Source: CAD feature listing. Evaluate the final solid. Frame: model axes, mm. Give positions to 0.01 mm unless a question says otherwise; leave off trailing zeros. Order: outer loops, then holes, each group sorted by start corner. A loop starts at its lowest first (then second) coordinate and runs counter-clockwise, first axis right, second up.
from build123d import *

# Parameters (mm, degrees)
ESQUISSE1_R                  = 4.1
ESQUISSE1_R_2                = 2.1
BOSS_EXTRU_1_DEPTH           = 6
ESQUISSE2_R                  = 17.5
BOSS_EXTRU_3_DEPTH           = 10
CONG_5_R                     = 0.5
R_P_TITION_CIRCULAIRE2_COUNT = 5
CONG_6_R                     = 0.5
ENL_V_MAT_EXTRU_1_DEPTH      = 1


with BuildPart() as part:
    # Esquisse1 → Boss.-Extru.1 (new body)
    with BuildSketch(Plane.XY):
        Circle(ESQUISSE1_R)
        Circle(ESQUISSE1_R_2, mode=Mode.SUBTRACT)
    extrude(amount=BOSS_EXTRU_1_DEPTH)

    # Esquisse2 → Boss.-Extru.3 (add)
    with BuildSketch(Plane.XY.offset(6)):
        Circle(ESQUISSE2_R)
        with BuildLine():
            Line((2, 3.579106034), (2, 15.370426149))
            ThreePointArc((2, 15.370426149), (0, -15.5), (-2, 15.370426149))
            Line((-2, 15.370426149), (-2, 3.579106034))
            ThreePointArc((-2, 3.579106034), (0, -4.1), (2, 3.579106034))
        make_face(mode=Mode.SUBTRACT)
        with BuildLine():
            Line((-0.5, 4.06939799), (-0.5, 15.491933385))
            ThreePointArc((-0.5, 15.491933385), (0, 15.5), (0.5, 15.491933385))
            Line((0.5, 15.491933385), (0.5, 4.06939799))
            ThreePointArc((0.5, 4.06939799), (0, 4.1), (-0.5, 4.06939799))
        make_face(mode=Mode.SUBTRACT)
    boss_extru_3 = extrude(amount=BOSS_EXTRU_3_DEPTH)

    # Congé5
    # the kernel refuses this fillet: 0.5 mm, written as the material it adds along each edge
    with BuildSketch(Plane(origin=(2, 3.579106034, 6), x_dir=(0.856640365534706, -0.5159140278540265, 0), z_dir=(0, 0, 1))) as cong_5_piece_1:
        with BuildLine():
            CenterArc((0.282708153, 0.499735946), CONG_5_R, 211.058569469, 57.079265472)
            Line((-0.14561203, 0.241778932), (0, 0))
            ThreePointArc((0, 0), (0.133230279, 0.002165243), (0.266460558, 0))
        make_face()
    extrude(amount=10)
    with BuildSketch(Plane(origin=(2, 15.370426149, 6), x_dir=(0, -1, 0), z_dir=(0, 0, 1))) as cong_5_piece_2:
        with BuildLine():
            CenterArc((0.580226691, 0.5), CONG_5_R, 170.405931773, 99.594068227)
            ThreePointArc((0.087220043, 0.583333333), (0.040835089, 0.292081575), (0, 0))
            Line((0, 0), (0.580226691, 0))
        make_face()
    extrude(amount=10)
    with BuildSketch(Plane(origin=(-2, 15.370426149, 6), x_dir=(0, -1, 0), z_dir=(0, 0, 1))) as cong_5_piece_3:
        with BuildLine():
            CenterArc((0.580226691, -0.5), CONG_5_R, 90, 99.594068227)
            ThreePointArc((0.087220043, -0.583333333), (0.040835089, -0.292081575), (0, 0))
            Line((0, 0), (0.580226691, 0))
        make_face()
    extrude(amount=10)
    with BuildSketch(Plane(origin=(-2, 3.579106034, 6), x_dir=(-0.8566403655347238, -0.515914027853997, 0), z_dir=(0, 0, 1))) as cong_5_piece_4:
        with BuildLine():
            CenterArc((0.282708153, -0.499735946), CONG_5_R, 91.862165059, 57.079265472)
            Line((-0.14561203, -0.241778932), (0, 0))
            ThreePointArc((0, 0), (0.133230279, -0.002165243), (0.266460558, 0))
        make_face()
    extrude(amount=10)

    # Répétition circulaire2: Boss.-Extru.3 ×5 about axis
    r_p_tition_circulaire2_axis = Axis((0, 0, 0), (0, 0, 1))
    for i in range(1, R_P_TITION_CIRCULAIRE2_COUNT):
        add(boss_extru_3.rotate(r_p_tition_circulaire2_axis, i * 360 / R_P_TITION_CIRCULAIRE2_COUNT))

    # Congé6
    # the kernel refuses this fillet: 0.5 mm, written as the material it adds along each edge
    with BuildSketch(Plane(origin=(-14.000109958, 6.651835923, 6), x_dir=(0.95105651629517, -0.3090169943748974, 0), z_dir=(0, 0, 1)), Plane(origin=(-10.652543801, -11.259365461, 6), x_dir=(0.5877852522924284, 0.8090169943749799, 0), z_dir=(0, 0, 1)), Plane(origin=(7.416475823, -13.61050647, 6), x_dir=(-0.5877852522925181, 0.8090169943749146, 0), z_dir=(0, 0, 1)), Plane(origin=(15.236177936, 2.847609858, 6), x_dir=(-0.9510565162951373, -0.30901699437499736, 0), z_dir=(0, 0, 1))) as cong_6_piece_1:
        with BuildLine():
            CenterArc((0.580226691, 0.5), CONG_6_R, 170.405931773, 99.594068227)
            ThreePointArc((0.087220043, 0.583333333), (0.040835089, 0.292081575), (0, 0))
            Line((0, 0), (0.580226691, 0))
        make_face()
    extrude(amount=10)
    with BuildSketch(Plane(origin=(-4.021966105, -0.796108444, 6), x_dir=(-0.9510565162951476, 0.30901699437496566, 0), z_dir=(0, 0, 1)), Plane(origin=(-0.485711754, -4.07112811, 6), x_dir=(-0.587785252292492, -0.8090169943749336, 0), z_dir=(0, 0, 1)), Plane(origin=(2.785898127, 3.008117622, 6), x_dir=(0.95105651629516, 0.30901699437492763, 0), z_dir=(0, 0, 1)), Plane(origin=(3.721779732, -1.719987101, 6), x_dir=(0.5877852522924618, -0.8090169943749556, 0), z_dir=(0, 0, 1))) as cong_6_piece_2:
        with BuildLine():
            CenterArc((0.282240882, 0.5), CONG_6_R, 212.920734528, 57.079265472)
            ThreePointArc((-0.13747074, 0.22826087), (-0.066880535, 0.115247514), (0, 0))
            Line((0, 0), (0.282240882, 0))
        make_face()
    extrude(amount=10)
    with BuildSketch(Plane(origin=(-2.785898127, 3.008117622, 6), x_dir=(-0.9510565162951584, 0.30901699437493263, 0), z_dir=(0, 0, 1)), Plane(origin=(0.485711754, -4.07112811, 6), x_dir=(0.5877852522924834, -0.80901699437494, 0), z_dir=(0, 0, 1)), Plane(origin=(4.021966105, -0.796108444, 6), x_dir=(0.9510565162951494, 0.3090169943749601, 0), z_dir=(0, 0, 1)), Plane(origin=(-3.721779732, -1.719987101, 6), x_dir=(-0.5877852522924625, -0.8090169943749551, 0), z_dir=(0, 0, 1))) as cong_6_piece_3:
        with BuildLine():
            CenterArc((0.282240882, -0.5), CONG_6_R, 90, 57.079265472)
            ThreePointArc((-0.13747074, -0.22826087), (-0.066880535, -0.115247514), (0, 0))
            Line((0, 0), (0.282240882, 0))
        make_face()
    extrude(amount=10)
    with BuildSketch(Plane(origin=(-15.236177936, 2.847609858, 6), x_dir=(0.9510565162950345, -0.3090169943753136, 0), z_dir=(0, 0, 1)), Plane(origin=(10.652543801, -11.259365461, 6), x_dir=(-0.5877852522921582, 0.8090169943751762, 0), z_dir=(0, 0, 1)), Plane(origin=(14.000109958, 6.651835923, 6), x_dir=(-0.9510565162952725, -0.30901699437458163, 0), z_dir=(0, 0, 1)), Plane(origin=(-7.416475823, -13.61050647, 6), x_dir=(0.5877852522927831, 0.8090169943747222, 0), z_dir=(0, 0, 1))) as cong_6_piece_4:
        with BuildLine():
            CenterArc((0.580226691, -0.5), CONG_6_R, 90, 99.594068227)
            ThreePointArc((0.087220043, -0.583333333), (0.040835089, -0.292081575), (0, 0))
            Line((0, 0), (0.580226691, 0))
        make_face()
    extrude(amount=10)

    # Esquisse3 → Enlèv. mat.-Extru.1 (cut)
    with BuildSketch(Plane.XY.offset(16)):
        with BuildLine():
            add(Edge.make_bspline(
                [(-0.781170014, 1.304004922), (-0.812563749, 1.155777067), (-0.779234347, 0.872861941), (-0.789120429, 0.435915264), (-0.779662215, 0.00403459), (-0.779566847, -0.436819947), (-0.790669805, -0.918125792), (-0.753886654, -1.254210502), (-0.812960802, -1.619629404), (-0.46848935, -1.526718543), (-0.210313129, -1.578712073), (0.206570231, -1.5215438), (0.483914566, -1.560659915), (0.894295895, -1.634559216), (0.820350644, -1.445502947), (0.844042185, -1.343660096), (0.813162572, -1.228475349), (0.936068838, -1.201220794), (1.049263647, -1.264408958), (1.196472414, -1.2143847), (1.354127977, -1.188939762), (1.48225229, -1.070899097), (1.630678619, -0.966920839), (1.756146104, -0.797993424), (1.747587013, -0.600658443), (1.793539651, -0.36734293), (1.705261694, -0.110947754), (1.73453965, 0.133450986), (1.698978601, 0.317241234), (1.675274487, 0.468699178), (1.567690497, 0.618342491), (1.350417168, 0.686766032), (1.143639018, 0.720499311), (0.9428535, 0.726655294), (0.85099379, 0.889975418), (0.8925264, 1.042820703), (0.861289404, 1.219750047), (0.912836482, 1.378714894), (0.792663409, 1.491607795), (0.638917577, 1.531180573), (0.440629112, 1.60203452), (0.20858732, 1.575087697), (-0.002645656, 1.564249374), (-0.193646565, 1.537998466), (-0.373102838, 1.592366964), (-0.539764419, 1.520975183), (-0.725989147, 1.491167171), (-0.768937119, 1.361763444), (-0.781170014, 1.304004922)],
                knots=[0, 0, 0, 0, 0.041401656, 0.082967656, 0.124831503, 0.16541839, 0.210270414, 0.259846062, 0.271899371, 0.299274831, 0.326037955, 0.357720778, 0.410942043, 0.427867114, 0.442662916, 0.451602915, 0.460542914, 0.470438204, 0.478266215, 0.497739299, 0.510942132, 0.523848972, 0.546138408, 0.563929013, 0.580743748, 0.601196424, 0.631542095, 0.655672873, 0.670757522, 0.685175475, 0.6992867, 0.721042554, 0.74732753, 0.762106015, 0.773798503, 0.795128896, 0.805353228, 0.825589214, 0.836672952, 0.847964087, 0.871314939, 0.896055832, 0.913792222, 0.932301035, 0.951146153, 0.96451384, 0.983867415, 1, 1, 1, 1], degree=3))
        make_face()
        with BuildLine():
            add(Edge.make_bspline(
                [(0.862853166, 0.319880005), (0.875242371, 0.203602803), (0.851846633, 0.015426685), (0.870814127, -0.293915634), (0.894410845, -0.55366391), (0.8562846, -0.775313723), (0.917218147, -1.002213112), (1.157109792, -0.996086818), (1.324288904, -0.917035516), (1.471649561, -0.796046729), (1.531405346, -0.606499314), (1.539582323, -0.393876838), (1.503758708, -0.19142601), (1.496156029, 0.000367913), (1.557995818, 0.217865985), (1.433984078, 0.472846391), (1.176337864, 0.505805782), (1.012207317, 0.545102616), (0.839476839, 0.465569349), (0.857164259, 0.373272475), (0.862853166, 0.319880005)],
                knots=[0, 0, 0, 0, 0.083463664, 0.157840166, 0.239391453, 0.285079185, 0.338278506, 0.392619199, 0.441520026, 0.487125232, 0.535865276, 0.591595143, 0.65293684, 0.696801833, 0.739973989, 0.83015049, 0.868591678, 0.937864877, 0.961674936, 1, 1, 1, 1], degree=3))
        make_face(mode=Mode.SUBTRACT)
    extrude(amount=-ENL_V_MAT_EXTRU_1_DEPTH, mode=Mode.SUBTRACT)


solid = part.part
(1) Section B-B, the plane y = -8. Return loops of the section in (x, z).
(2) Section C-C, the plane z = 13. Count the separate pieces of the cut face and the enclosed holes in it, plus the area to 3 significant figures.
(3) Section A-A, the plane y = 14. Return loops of the section in (x, z), plus the area to 3 significant figures.
(4) Draft query along X for faces 1 (the flat face through (-1.5, -4.9, 6)), 2 (the flat face through (9.415, 0.956, 10.93)). Return one class per face: +X half, -X half, draft (parallel to the pull), parting line (faces both ways), or undercut.
(5) Pin query (flat end, axial travel): pin 1 Ø8 at (y, z) = (9.5, 10.5) entering from +X; pin 2 Ø8 at (y, z) = (7.5, 12) entering from -X; pin 3 Ø3 at (y, z) = (10, 10) entering from +X. Return the tip coordinate at first contact, or that it passes through.
(6) Section D-D, the plane z = 4.5. Return loops of the section in (x, y).
(7) Line query: line 1 along X through (y, z) = (-5.5, 8.5); line 2 along X through (y, z) = (13, 11.75); line 3 along Y through (x, z) = (0, 3.8). Output: solid intervals per line, ascending.
Checks:
1. outline: (-15.56, 6) - (-13.28, 6) - (-13.28, 16) - (-15.56, 16) - close; (-8.28, 6) - (-6.43, 6) - (-6.43, 16) - (-8.28, 16) - close; (-5.19, 6) - (-3.34, 6) - (-3.34, 16) - (-5.19, 16) - close; (3.34, 6) - (5.19, 6) - (5.19, 16) - (3.34, 16) - close; (6.43, 6) - (8.28, 6) - (8.28, 16) - (6.43, 16) - close; (13.28, 6) - (15.56, 6) - (15.56, 16) - (13.28, 16) - close
2. separate pieces: 1
2. enclosed holes: 10
2. area: 435 mm2
3. outline: (-10.5, 6) - (-6.65, 6) - (-6.65, 16) - (-10.5, 16) - close; (-2, 6) - (-0.5, 6) - (-0.5, 16) - (-2, 16) - close; (0.5, 6) - (2, 6) - (2, 16) - (0.5, 16) - close; (6.65, 6) - (10.5, 6) - (10.5, 16) - (6.65, 16) - close
3. area: 107 mm2
4. face 1: draft
4. face 2: undercut
5. pin 1: stops at x = 16.61
5. pin 2: stops at x = -17.15
5. pin 3: stops at x = 15.3
6. outline: circle Ø8.2 at (0, 0); hole circle Ø4.2 at (0, 0)
7. line 1: x = -16.61 to -14.49, -6.47 to -4.61, -3.38 to -1.52, 1.52 to 3.38, 4.61 to 6.47, 14.49 to 16.61
7. line 2: x = -11.72 to -8.44, -2 to -0.5, 0.5 to 2, 8.44 to 11.72
7. line 3: y = -4.1 to -2.1, 2.1 to 4.1
